```python
from build123d import *

# Parameters (mm, degrees)
F3_SIZE = 0.5
F5_D    = 3.3


with BuildPart() as f1:
    # F0 (on Front) → F1 (revolve)
    with BuildSketch(Plane.XZ):
        Polygon((0, 3.6), (0, 0), (40, 0), (40, 4.9), (20, 4.9), (20, 10), (-40, 10), (-40, 5.05), (-20, 5.05), (-20, 3.6), align=None)
    revolve(axis=Axis((-1.4153197408, 0, 0), (1, 0, 0)))

    # F3
    f3_edges = [f1.edges().sort_by_distance(p)[0] for p in [
        (-40, 0, -10),
        (40, 0, -4.9),
    ]]
    chamfer(f3_edges, length=F3_SIZE)

    # F5 (through all)
    with Locations(Plane(origin=(0, 0, -25), x_dir=(1, 0, 0), z_dir=(0, 0, -1))):
        with Locations((-15, 0), (-3, 0)):
            Hole(F5_D / 2)


solid = f1.part
```
Source: CAD feature listing. Evaluate the final solid. Frame: model axes, mm. A direction names the side the tool comes from. Round coordinates to 2 decimals unless told otherwise and drop trailing zeros. Write each loop counter-clockwise with the first axis right and the second up, starting at its lowest first coordinate (ties: lowest second). Pieces come first, ordered by that corner, then holes. Notation, with made-up numbers: M 42.25,-37 L 64.25,-37 A25 ccw 64.25,-7 Z; hole C -16.75,78 d5. An arc over 180 degrees is marked long. Answer as a JSON object with one key per item and string values. Group by question number.
(1) Ray query, line 1 (X direction, y = 1.5, z = -2.75); line 2 (Y direction, x = -34.75, z = 0); line 3 (Y direction, x = -14.75, z = 0). Return the intervals inside material, ascending. Write a range as [from, to].
(2) Section query C-C on x = -15. Output: boundary loops of the cut face in (y, z), then the cut area to 3 significant figures.
(3) Section query D-D on x = 33. Output: boundary loops of the cut face in (y, z).
(4) Mould query, pull axis X, two halves, no side actions, for faces 1 (the flat face through (0, 0, 0)), 2 (the cylindrical face through (-1.35, -0.07, 6.65)), 3 (the cylindrical face through (-29.86, -1.517, 4.817)), 4 (the cylindrical face through (-1.35, -0.07, -6.55)). Classes: +X half, -X half, draft (parallel to the pull), parting line (faces both ways), or undercut.
(5) Section query A-A on z = 0. Output: boundary loops of the cut face in (x, y).
(6) Reachability of faces 5 (the cylindrical face through (29.614, 4.783, -1.062)), 6 (the flat face through (-40, 4, 4)), 7 (the cylindrical face through (-9.86, -0.158, -3.597)) from +Z, -Z, +X, -X, +Y, -Y: full face, straight path, thin tool, end or side. Return the list, or none.
(7) Section query B-B on y = 0. State how many separate pieces and enclosed holes the cut face has, then the cut area to 3 significant figures.
(8) First-contact query: pin 1 (1.5 mm diameter, centred on x = 12, z = 5, fed in from +Y); pin 2 (2 mm diameter, centred on x = -15, y = 0, fed in from -Z); pin 3 (6 mm diameter, centred on y = 0, z = 0, fed in from -X); pin 4 (4 mm diameter, centred on x = -1.5, z = -2.5, fed in from -Y). Flat tips, straight axial feed; report the tip coordinate or a pass-through.
Computed values:
{
 "1": {"line 1": "[0, 40]", "line 2": "[-10, -5.05], [5.05, 10]", "line 3": "[-10, -3.6], [3.6, 10]"},
 "2": {"outline": "M -1.65,-9.86 L -1.65,-3.2 A3.6 cw -1.65,3.2 L -1.65,9.86 A10 ccw Z; M 1.65,-9.86 A10 ccw 1.65,9.86 L 1.65,3.2 A3.6 cw 1.65,-3.2 Z", "area": "231 mm^2"},
 "3": {"outline": "C 0,0 d9.8"},
 "4": {"face 1": "-X half", "face 2": "undercut", "face 3": "draft", "face 4": "undercut"},
 "5": {"outline": "M -40,-9.5 L -39.5,-10 L 20,-10 L 20,-4.9 L 39.5,-4.9 L 40,-4.4 L 40,4.4 L 39.5,4.9 L 20,4.9 L 20,10 L -39.5,10 L -40,9.5 L -40,5.05 L -20,5.05 L -20,3.6 L 0,3.6 L 0,-3.6 L -20,-3.6 L -20,-5.05 L -40,-5.05 Z"},
 "6": {"face 5": "+X", "face 6": "+Z, -Z, -X, +Y, -Y", "face 7": "-X"},
 "7": {"separate pieces": "5", "enclosed holes": "0", "area": "965 mm^2"},
 "8": {"pin 1": "y = 9.05", "pin 2": "through", "pin 3": "x = 0", "pin 4": "y = -9.99"}
}
